```python
from build123d import *

# Parameters (mm, degrees)
F0_R      = 1.5320214601
F1_DEPTH  = 4.8
F0_R_2    = 2.5
F2_DEPTH  = 3.9
F4_DEPTH  = 2.5
F6_DEPTH  = 2.5
F7_DEPTH  = 3.2
F8_W      = 0.2057314705
F8_H      = 0.1714428654
F9_DEPTH  = 0.4
F11_DEPTH = 0.25
F12_DEPTH = 0.43


with BuildPart() as f1:
    # F0 (on Top) → F1 (new body, symmetric)
    with BuildSketch(Plane.XY):
        Circle(F0_R)
        Polygon((0.039557572, 1.1622756139), (1.1176137583, 0.3215414302), (0.6511657169, -0.9635520812), (-0.715171213, -0.9170493663), (-1.0931658343, 0.3967844035), align=None, mode=Mode.SUBTRACT)
    extrude(amount=F1_DEPTH, both=True)

    # F0 (on Top) → F2 (join, symmetric)
    with BuildSketch(Plane.XY):
        Circle(F0_R_2)
        Circle(F0_R, mode=Mode.SUBTRACT)
    extrude(amount=F2_DEPTH, both=True)

    # F3 (on Front) → F4 (join, symmetric)
    with BuildSketch(Plane.XZ):
        Polygon((2.4489383213, 2.6739891618), (0, 2.6739891618), (1.5983604826, 0.8004051051), align=None)
        Polygon((-1.5983604826, 0.8004051051), (0, 2.6739891618), (-2.4489383213, 2.6739891618), align=None)
        Polygon((0, 0), (0, 2.6739891618), (-1.5983604826, 0.8004051051), (-1.5983604826, 0), align=None)
        Polygon((1.5983604826, 0.8004051051), (0, 2.6739891618), (0, 0), (1.5983604826, 0), align=None)
        Polygon((2.2811886085, 0), (1.5983604826, 0.8004051051), (1.5983604826, 0), (1.5983604826, -0.8004051051), align=None)
        Polygon((-1.5983604826, 0), (-1.5983604826, 0.8004051051), (-2.2811886085, 0), (-1.5983604826, -0.8004051051), align=None)
        Polygon((0, -2.6739891618), (0, 0), (-1.5983604826, 0), (-1.5983604826, -0.8004051051), align=None)
        Polygon((1.5983604826, 0), (0, 0), (0, -2.6739891618), (1.5983604826, -0.8004051051), align=None)
        Polygon((1.5983604826, -0.8004051051), (0, -2.6739891618), (2.4489383213, -2.6739891618), align=None)
        Polygon((-2.4489383213, -2.6739891618), (0, -2.6739891618), (-1.5983604826, -0.8004051051), align=None)
    extrude(amount=F4_DEPTH, both=True)

    # F5 (on Right) → F6 (join, symmetric)
    with BuildSketch(Plane.YZ):
        Polygon((1.4358381741, 0.9031511727), (0, 2.7375903446), (-1.4358381741, 0.9031511727), (-0.5977854705, 0.2471969813), (-1.4358381741, -1.0170094902), (-0.5977854705, -2.3199757561), (0.5977854705, -2.3199757561), (1.4358381741, -1.0170094902), (0.5977854705, 0.2471969813), align=None)
    extrude(amount=F6_DEPTH, both=True)

    # F7 (cut): a face of the model
    f7_faces = [f1.faces().sort_by_distance(p)[0] for p in [
        (-1.4886893496, 0, 4.8),
    ]]
    extrude(f7_faces, amount=-F7_DEPTH, mode=Mode.SUBTRACT)

    # F8 (on face) → F9 (join)
    with BuildSketch(Plane.XZ.offset(2.5)):
        Polygon((-0.181210431, -0.4586814321), (-0.181210431, -1.0104251851), (1.1774745134, -1.0104251851), (1.4746332308, -0.7784541231), (1.1832588352, -0.7784541231), (0.7335068658, -0.7784541231), (0.7335068658, -0.4586814321), (0.4220934934, -0.4586814321), (0.4220934934, -0.7784541231), (0.1979402587, -0.7784541231), (0.1979402587, -0.4586814321), align=None)
        Polygon((0, 1.6032253625), (0, 1.8050573999), (-1.0815345449, 1.8050573999), (-1.0815345449, 1.6032253625), (-0.5499689287, 1.6032253625), (-0.5499689287, 1.1543665896), (0, 1.1543665896), align=None)
        with Locations((-0.2835566193, 1.4216544223)):
            Rectangle(F8_W, F8_H, mode=Mode.SUBTRACT)
        Polygon((0.5908022868, 1.8074008403), (0.5908022868, 1.2759278761), (1.2337132357, 1.2759278761), (1.6023155767, 1.2759278761), (1.6023155767, 1.7541147536), (1.5667511437, 1.7541147536), (1.529708039, 1.7541147536), (1.529708039, 1.3383656042), (1.1996804969, 1.3380937204), (1.0839564493, 1.3379983845), (1.0839564493, 1.8074008403), (1.0386969661, 1.8074008403), (1.0386969661, 1.4045101125), (0.8136780816, 1.4045101125), (0.8136780816, 1.8074008403), align=None)
        Polygon((0.7572061731, 1.7627113266), (0.7572061731, 1.3381995394), (0.6472741952, 1.3391206739), (0.6472741952, 1.7627113266), align=None, mode=Mode.SUBTRACT)
        Polygon((1.5667511437, 1.7541147536), (1.6023155767, 1.7541147536), (1.6023155767, 1.8074008403), (1.4394447207, 1.8074008403), (1.4394447207, 1.7541147536), (1.529708039, 1.7541147536), align=None)
        Polygon((1.529708039, 1.3383656042), (1.529708039, 1.7541147536), (1.4394447207, 1.7541147536), (1.4394447207, 1.4045101125), (1.2337132357, 1.4045101125), (1.2337132357, 1.8074008403), (1.1996804969, 1.8074008403), (1.1996804969, 1.3380937204), align=None)
        Polygon((1.1996804969, 1.8074008403), (1.0839564493, 1.8074008403), (1.0839564493, 1.3379983845), (1.1996804969, 1.3380937204), align=None)
    extrude(amount=F9_DEPTH)

    # F10 (on Right) → F11 (join, symmetric)
    with BuildSketch(Plane.YZ):
        Polygon((0, 10.4586472735), (0, 3.8638201077), (1.8880540525, 3.8153284695), (1.8880540525, 10.4586472735), (5.5842293836, 13.2371469554), (4.9025323242, 14.1439931467), align=None)
        Polygon((1.8880540525, -3.8153284695), (0, -3.8638201077), (0, -10.4586472735), (4.9025323242, -14.1439931467), (5.5842293836, -13.2371469554), (1.8880540525, -10.4586472735), align=None)
    extrude(amount=F11_DEPTH, both=True)

    # F8 (on face) → F12 (join)
    with BuildSketch(Plane.XZ.offset(2.5)):
        Polygon((-0.181210431, -0.4586814321), (-0.181210431, -1.0104251851), (1.1774745134, -1.0104251851), (1.4746332308, -0.7784541231), (1.1832588352, -0.7784541231), (0.7335068658, -0.7784541231), (0.7335068658, -0.4586814321), (0.4220934934, -0.4586814321), (0.4220934934, -0.7784541231), (0.1979402587, -0.7784541231), (0.1979402587, -0.4586814321), align=None)
        Polygon((0, 1.6032253625), (0, 1.8050573999), (-1.0815345449, 1.8050573999), (-1.0815345449, 1.6032253625), (-0.5499689287, 1.6032253625), (-0.5499689287, 1.1543665896), (0, 1.1543665896), align=None)
        with Locations((-0.2835566193, 1.4216544223)):
            Rectangle(F8_W, F8_H, mode=Mode.SUBTRACT)
        Polygon((0.5908022868, 1.8074008403), (0.5908022868, 1.2759278761), (1.2337132357, 1.2759278761), (1.6023155767, 1.2759278761), (1.6023155767, 1.7541147536), (1.5667511437, 1.7541147536), (1.529708039, 1.7541147536), (1.529708039, 1.3383656042), (1.1996804969, 1.3380937204), (1.0839564493, 1.3379983845), (1.0839564493, 1.8074008403), (1.0386969661, 1.8074008403), (1.0386969661, 1.4045101125), (0.8136780816, 1.4045101125), (0.8136780816, 1.8074008403), align=None)
        Polygon((0.7572061731, 1.7627113266), (0.7572061731, 1.3381995394), (0.6472741952, 1.3391206739), (0.6472741952, 1.7627113266), align=None, mode=Mode.SUBTRACT)
        Polygon((1.5667511437, 1.7541147536), (1.6023155767, 1.7541147536), (1.6023155767, 1.8074008403), (1.4394447207, 1.8074008403), (1.4394447207, 1.7541147536), (1.529708039, 1.7541147536), align=None)
        Polygon((1.529708039, 1.3383656042), (1.529708039, 1.7541147536), (1.4394447207, 1.7541147536), (1.4394447207, 1.4045101125), (1.2337132357, 1.4045101125), (1.2337132357, 1.8074008403), (1.1996804969, 1.8074008403), (1.1996804969, 1.3380937204), align=None)
        Polygon((1.1996804969, 1.8074008403), (1.0839564493, 1.8074008403), (1.0839564493, 1.3379983845), (1.1996804969, 1.3380937204), align=None)
    extrude(amount=F12_DEPTH)


solid = f1.part
```
Geometry: final body of the model. Coordinates: model frame, mm. A direction names the side the tool comes from. Round coordinates to 2 decimals unless told otherwise and drop trailing zeros. Write each loop counter-clockwise with the first axis right and the second up, starting at its lowest first coordinate (ties: lowest second). Pieces come first, ordered by that corner, then holes. Notation, with made-up numbers: M 44.5,-21.75 L 75.5,-21.75 A18 cw 75.5,1.25 Z; hole C -23,46.5 d7. An arc over 180 degrees is marked long. Answer in a Markdown table with one row per item. Add a question column.
(1) Draft query along Z for faces 5 (the face through (2.11, 1.93, 1.93)), 6 (the face through (0, -0.5, 2.674)). Return one class per face: pulls with the +Z half, pulls with the -Z half, needs draft (parallel to the pull), parting line crosses it, or undercut.
(2) Cut plane B-B, the plane z = 9. Return the cut outline in (x, y), then the cut area to 3 significant figures.
(3) Reachability of faces 1 (the face through (-2.11, 1.93, -1.93)), 2 (the face through (-2, -2, 2.674)), 3 (the face through (2.02, -1.936, 0.306)), 4 (the face through (2.02, 1.915, 0.306)) from +Z, -Z, +X, -X, +Y, -Y: full face, straight path, thin tool, end or side. Return the list, or none.
(4) Cut plane A-A, the plane y = 3.25. Return the cut outline in (x, z), then the cut area to 3 significant figures.
(5) Ray query, L1, parallel to Y at x = 0, z = 3.1; L2, parallel to Z at x = 2.1, y = -2. Return the intervals inside material, ascending.
(6) Contact query for flat-ended pins moving along their axis: pin 1 (1 mm diameter, centred on x = 1.5, y = 1.5, fed in from +Z); pin 2 (3 mm diameter, centred on x = -0.5, z = -6.5, fed in from +Y); pin 3 (4.5 mm diameter, centred on y = 4, z = 9.5, fed in from +X); pin 4 (3 mm diameter, centred on y = 4, z = 9, fed in from -X). Output: stop coordinate, or through.
Established:
| question | item | result |
|---|---|---|
| 1 | face 5 | undercut |
| 1 | face 6 | pulls with the +Z half |
| 2 | outline | M -0.25,0 L 0.25,0 L 0.25,1.89 L -0.25,1.89 Z |
| 2 | area | 0.944 mm² |
| 3 | face 1 | -X, +Y |
| 3 | face 2 | +Z, -X, -Y |
| 3 | face 3 | +X, -Y |
| 3 | face 4 | +X, +Y |
| 4 | outline | M -0.25,-12.9 L 0.25,-12.9 L 0.25,-11.48 L -0.25,-11.48 Z; M -0.25,11.48 L 0.25,11.48 L 0.25,12.9 L -0.25,12.9 Z |
| 4 | area | 1.42 mm² |
| 5 | L1 | -2.5 to -1.53, 1.53 to 2.5 |
| 5 | L2 | -2.67 to -1.91, -0.21 to 0.21, 1.91 to 2.67 |
| 6 | pin 1 | z = 3.9 |
| 6 | pin 2 | y = 1.89 |
| 6 | pin 3 | x = 0.25 |
| 6 | pin 4 | through |
